Geometry: see drawing. Coordinates: mm, zero at the bounding-box minimum. Give positions to 0.01 mm unless a question says otherwise; leave off trailing zeros. Order: outer loops, then holes, each group sorted by start corner. A loop starts at its lowest first (then second) coordinate and runs counter-clockwise, first axis right, second up. Notation, with made-up numbers: M -35,87.5 L -30,87.5 A37 ccw -30,123.5 Z; hole C 32.5,13 d5. An arc over 180 degrees is marked long. Write item = value, one per line. Start each with the question number.
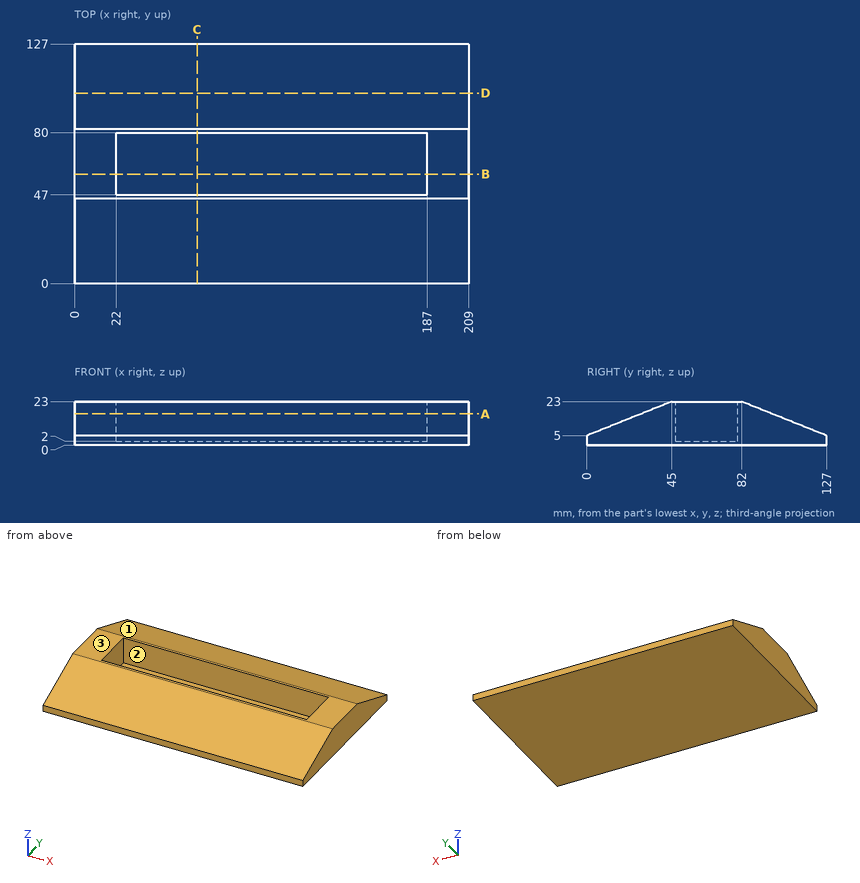
1) Ray query, L1, parallel to X at y = 63.5, z = 10; L2, parallel to Z at x = 153, y = 72; L3, parallel to Z at x = 123, y = 37.5. Return the intervals inside material, ascending.
2) Cut plane C-C (x = 65). Return loops of the section in (y, z), plus the area to 3 significant figures.
3) Cut plane D-D (y = 101). Return loops of the section in (x, z).
4) Pin query (flat end, axial travel): pin 1 Ø5 at (x, z) = (118, 10.5) entering from -Y; pin 2 Ø16.5 at (x, y) = (140, 62.5) entering from +Z; pin 3 Ø5 at (x, y) = (134, 100) entering from +Z. Return the tip coordinate at first contact, or that it passes through.
5) Cut plane B-B (y = 58). Return loops of the section in (x, z).
6) Draft query along Y for the marked faces 1, 2 and 3. Return one class per face: pulls with the +Y half, pulls with the -Y half, needs draft (parallel to the pull), parting line crosses it, or undercut.
7) Cut plane A-A (z = 16.5). Return loops of the section in (x, y), plus the area to 3 significant figures.
Reply:
q1.L1 = 0 to 22, 187 to 209
q1.L2 = 0 to 2
q1.L3 = 0 to 20
q2.outline = M 0,0 L 127,0 L 127,5 L 82,23 L 80,23 L 80,2 L 47,2 L 47,23 L 45,23 L 0,5 Z
q2.area = 1,420 mm²
q3.outline = M 0,0 L 209,0 L 209,15.4 L 0,15.4 Z
q4.pin_1 = 7.5
q4.pin_2 = 2
q4.pin_3 = 16.8
q5.outline = M 0,0 L 209,0 L 209,23 L 187,23 L 187,2 L 22,2 L 22,23 L 0,23 Z
q6.face_1 = pulls with the +Y half
q6.face_2 = undercut
q6.face_3 = needs draft
q7.outline = M 0,28.75 L 209,28.75 L 209,98.25 L 0,98.25 Z; hole M 22,47 L 187,47 L 187,80 L 22,80 Z
q7.area = 9,080 mm²
